Answer from the drawing. Dimensions are ordinates in mm from the lowest x, y and z of the part. Round coordinates to 2 decimals unless told otherwise and drop trailing zeros. Loops run counter-clockwise (first coordinate to the right, second up) from the corner with the lowest first, then second, coordinate; pieces in that order, holes last. Notation, with made-up numbers: M 86,75 L 140,75 A10 cw 140,91 Z; hole C 19.5,-39 d7. An arc over 180 degrees is marked long. Answer as a JSON object with one key per item and string values.
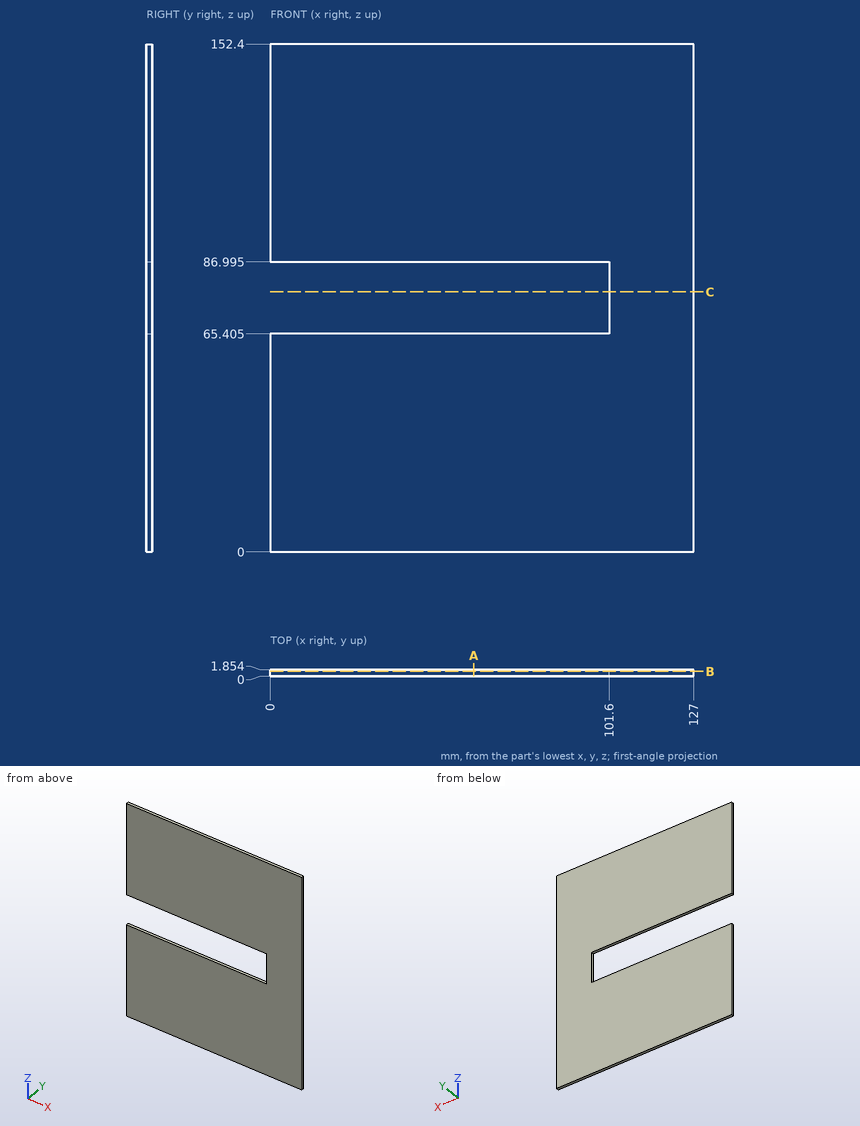
Item 1: The part is cut by section C-C (z = 78). Give the vertices of the cut face in (x, y).
Values follow:
{"outline": "M 101.6,0 L 127,0 L 127,1.85 L 101.6,1.85 Z"}
Item 2: The part is cut by section A-A (x = 61). Give the vertices of the cut face in (y, z) (1 decimal).
Values follow:
{"outline": "M 0,0 L 1.9,0 L 1.9,65.4 L 0,65.4 Z; M 0,87 L 1.9,87 L 1.9,152.4 L 0,152.4 Z"}
Item 3: The part is cut by section B-B (y = 1.4). Give the vertices of the cut face in (x, z) (3 decimals).
Values follow:
{"outline": "M 0,0 L 127,0 L 127,152.4 L 0,152.4 L 0,86.995 L 101.6,86.995 L 101.6,65.405 L 0,65.405 Z"}
Item 4: Straight lines are drawn through the part: line 1 (Z direction, x = 45.5, y = 1.55) (3 decimals); line 2 (X direction, y = 0.7, z = 79). For each, find the intervals that lie inside material, in ascending order.
Values follow:
{"line 1": "0 to 65.405, 86.995 to 152.4", "line 2": "101.6 to 127"}
